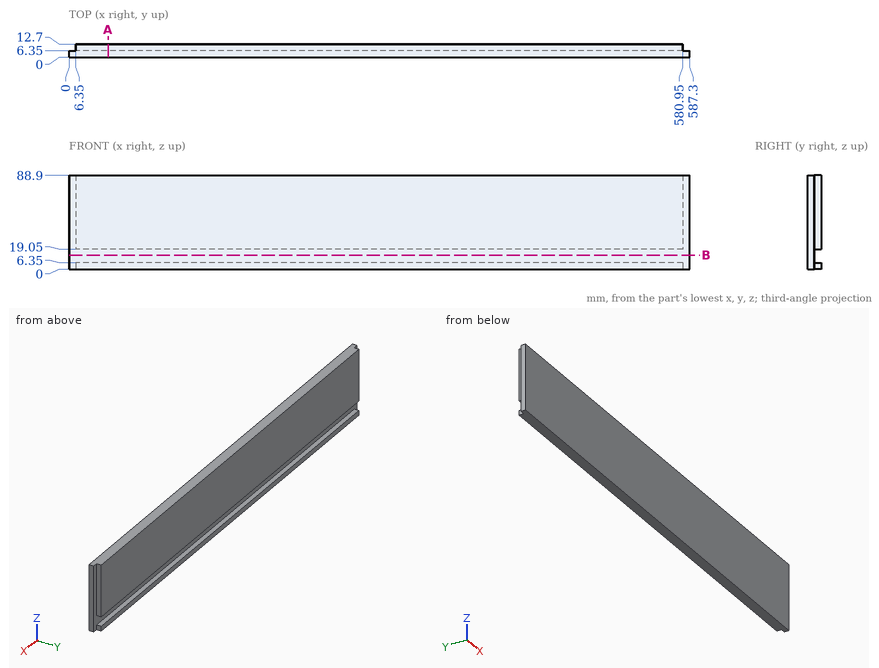
The figure shows three views and two pictorial views of one solid part (mm, origin at its lowest corner). Answer the questions. Coordinates: 2 decimals unless noted, no trailing zeros. Loops run counter-clockwise (first coordinate to the right, second up) from the corner with the lowest first, then second, coordinate; pieces in that order, holes last. Notation, with made-up numbers: (-27.75, 28.5) - (-11.75, 28.5) arc R17 ccw to (-11.75, 49.5) - close; hole circle Ø1 at (62.5, 82.5). An arc over 180 degrees is marked (long way). Use a Markdown table: item, result. Add a question column.
1) Find the intervals of material crossed by line 1 (Z direction, x = 335, y = 9.5); line 2 (X direction, y = 11.25, z = 83); line 3 (Y direction, x = 560.5, z = 14.5), in increasing order.
2) Given pin 1 (5 mm diameter, centred on y = 8.5, z = 4.5, fed in from -X); pin 2 (3 mm diameter, centred on y = 9.5, z = 27, fed in from -X); pin 3 (1 mm diameter, centred on x = 327, z = 11, fed in from +Y); pin 4 (7 mm diameter, centred on y = 10.5, z = 45.5, fed in from +X), each flat-ended and moving along its own axis, determine where each tip first touches the part or whether it passes through.
3) The part is cut by section A-A, the plane x = 37. Give the vertices of the cut face in (y, z).
4) The part is cut by section B-B, the plane z = 13.5. Give the vertices of the cut face in (x, y).
Here are the results:
| question | item | result |
|---|---|---|
| 1 | line 1 | z = 0 to 6.35, 19.05 to 88.9 |
| 1 | line 2 | x = 6.35 to 580.95 |
| 1 | line 3 | y = 0 to 6.35 |
| 2 | pin 1 | stops at x = 0 |
| 2 | pin 2 | stops at x = 6.35 |
| 2 | pin 3 | stops at y = 6.35 |
| 2 | pin 4 | stops at x = 580.95 |
| 3 | outline | (0, 0) - (12.7, 0) - (12.7, 6.35) - (6.35, 6.35) - (6.35, 19.05) - (12.7, 19.05) - (12.7, 88.9) - (0, 88.9) - close |
| 4 | outline | (0, 0) - (587.3, 0) - (587.3, 6.35) - (0, 6.35) - close |
